from build123d import *

# Parameters (mm, degrees)
F0_R     = 2.50825
F1_DEPTH = 1.5875
F2_R     = 1.27


with BuildPart() as f1:
    # F0 (on Top) → F1 (new body)
    with BuildSketch(Plane.XY):
        with BuildLine():
            Line((2.667, 95.25), (0, 95.25))
            Line((0, 95.25), (-2.667, 95.25))
            ThreePointArc((-2.667, 95.25), (-3.5342102448, 94.8907897552), (-3.175, 95.758))
            Line((-3.175, 95.758), (-3.175, 114.3))
            Line((-3.175, 114.3), (-24.765, 114.3))
            Line((-24.765, 114.3), (-24.765, 0))
            Line((-24.765, 0), (-5.2613402643, -16.3655136908))
            ThreePointArc((-5.2613402643, -16.3655136908), (-3.9082748076, -16.5436481376), (-3.175, -15.3926372481))
            Line((-3.175, -15.3926372481), (-3.175, -0.508))
            ThreePointArc((-3.175, -0.508), (-3.5342102448, 0.3592102448), (-2.667, 0))
            Line((-2.667, 0), (0, 0))
            Line((0, 0), (2.667, 0))
            ThreePointArc((2.667, 0), (3.3487462328, 0.4773638514), (3.5641505771, -0.3265361057))
            ThreePointArc((3.5641505771, -0.3265361057), (3.389690077, -0.4604043558), (3.175, -0.508))
            Line((3.175, -0.508), (3.175, -15.3926372481))
            ThreePointArc((3.175, -15.3926372481), (3.9082748076, -16.5436481376), (5.2613402643, -16.3655136908))
            Line((5.2613402643, -16.3655136908), (24.765, 0))
            Line((24.765, 0), (24.765, 114.3))
            Line((24.765, 114.3), (3.175, 114.3))
            Line((3.175, 114.3), (3.175, 95.758))
            ThreePointArc((3.175, 95.758), (3.5342102448, 94.8907897552), (2.667, 95.25))
        make_face()
        with BuildLine():
            ThreePointArc((-3.683, 17.8998578738), (-3.175, 18.4078578738), (-2.667, 17.8998578738))
            Line((-2.667, 17.8998578738), (-2.667, 10.2798578738))
            ThreePointArc((-2.667, 10.2798578738), (-3.175, 9.7718578738), (-3.683, 10.2798578738))
            Line((-3.683, 10.2798578738), (-3.683, 17.8998578738))
        make_face(mode=Mode.SUBTRACT)
        with BuildLine():
            ThreePointArc((-3.683, 34.8687778738), (-3.175, 35.3767778738), (-2.667, 34.8687778738))
            Line((-2.667, 34.8687778738), (-2.667, 27.2487778738))
            ThreePointArc((-2.667, 27.2487778738), (-3.175, 26.7407778738), (-3.683, 27.2487778738))
            Line((-3.683, 27.2487778738), (-3.683, 34.8687778738))
        make_face(mode=Mode.SUBTRACT)
        with BuildLine():
            Line((-3.683, 44.2176978738), (-3.683, 51.8376978738))
            ThreePointArc((-3.683, 51.8376978738), (-3.175, 52.3456978738), (-2.667, 51.8376978738))
            Line((-2.667, 51.8376978738), (-2.667, 44.2176978738))
            ThreePointArc((-2.667, 44.2176978738), (-3.175, 43.7096978738), (-3.683, 44.2176978738))
        make_face(mode=Mode.SUBTRACT)
        with BuildLine():
            Line((3.683, 17.8998578738), (3.683, 10.2798578738))
            ThreePointArc((3.683, 10.2798578738), (3.175, 9.7718578738), (2.667, 10.2798578738))
            Line((2.667, 10.2798578738), (2.667, 17.8998578738))
            ThreePointArc((2.667, 17.8998578738), (3.175, 18.4078578738), (3.683, 17.8998578738))
        make_face(mode=Mode.SUBTRACT)
        with BuildLine():
            Line((3.683, 34.8687778738), (3.683, 27.2487778738))
            ThreePointArc((3.683, 27.2487778738), (3.175, 26.7407778738), (2.667, 27.2487778738))
            Line((2.667, 27.2487778738), (2.667, 34.8687778738))
            ThreePointArc((2.667, 34.8687778738), (3.175, 35.3767778738), (3.683, 34.8687778738))
        make_face(mode=Mode.SUBTRACT)
        with BuildLine():
            Line((3.683, 51.8376978738), (3.683, 44.2176978738))
            ThreePointArc((3.683, 44.2176978738), (3.175, 43.7096978738), (2.667, 44.2176978738))
            Line((2.667, 44.2176978738), (2.667, 51.8376978738))
            ThreePointArc((2.667, 51.8376978738), (3.175, 52.3456978738), (3.683, 51.8376978738))
        make_face(mode=Mode.SUBTRACT)
        with BuildLine():
            ThreePointArc((-3.683, 68.8048978738), (-3.175, 69.3128978738), (-2.667, 68.8048978738))
            Line((-2.667, 68.8048978738), (-2.667, 61.1848978738))
            ThreePointArc((-2.667, 61.1848978738), (-3.175, 60.6768978738), (-3.683, 61.1848978738))
            Line((-3.683, 61.1848978738), (-3.683, 68.8048978738))
        make_face(mode=Mode.SUBTRACT)
        with Locations((-12.7, 104.775)):
            Circle(F0_R, mode=Mode.SUBTRACT)
        with BuildLine():
            ThreePointArc((-3.683, 85.7720978738), (-3.175, 86.2800978738), (-2.667, 85.7720978738))
            Line((-2.667, 85.7720978738), (-2.667, 78.1520978738))
            ThreePointArc((-2.667, 78.1520978738), (-3.175, 77.6440978738), (-3.683, 78.1520978738))
            Line((-3.683, 78.1520978738), (-3.683, 85.7720978738))
        make_face(mode=Mode.SUBTRACT)
        with BuildLine():
            Line((3.683, 68.8048978738), (3.683, 61.1848978738))
            ThreePointArc((3.683, 61.1848978738), (3.175, 60.6768978738), (2.667, 61.1848978738))
            Line((2.667, 61.1848978738), (2.667, 68.8048978738))
            ThreePointArc((2.667, 68.8048978738), (3.175, 69.3128978738), (3.683, 68.8048978738))
        make_face(mode=Mode.SUBTRACT)
        with BuildLine():
            Line((3.683, 85.7720978738), (3.683, 78.1520978738))
            ThreePointArc((3.683, 78.1520978738), (3.175, 77.6440978738), (2.667, 78.1520978738))
            Line((2.667, 78.1520978738), (2.667, 85.7720978738))
            ThreePointArc((2.667, 85.7720978738), (3.175, 86.2800978738), (3.683, 85.7720978738))
        make_face(mode=Mode.SUBTRACT)
        with Locations((12.7, 104.775)):
            Circle(F0_R, mode=Mode.SUBTRACT)
    extrude(amount=F1_DEPTH)

    # F2
    f2_edges = [f1.edges().sort_by_distance(p)[0] for p in [
        (24.765, 0, 0.79375),
        (-24.765, 0, 0.79375),
        (-24.765, 114.3, 0.79375),
        (24.765, 114.3, 0.79375),
    ]]
    fillet(f2_edges, radius=F2_R)


solid = f1.part
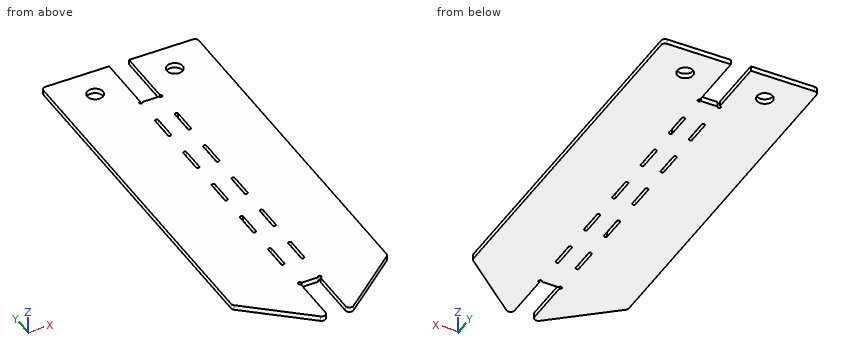
The listing builds one solid part. Answer for the finished solid, in the listing's coordinates (mm). Give positions to 0.01 mm unless a question says otherwise; leave off trailing zeros. Write each loop counter-clockwise with the first axis right and the second up, starting at its lowest first coordinate (ties: lowest second). Pieces come first, ordered by that corner, then holes.
1) Given P1, Ø6, axis at x = 12.7, y = 104.775, coming from the -Z side; P2, Ø0.9, axis at x = 3.175, y = 0, coming from the -Z side, each flat-ended and moving along its own axis, determine where each tip first touches the part or whether it passes through.
2) Section B-B (x = -12.7) is taken. Write down the section's boundary in (y, z), and give its area (3 significant figures).
3) Find the intervals of material crossed by L1, parallel to X at y = 85, z = 0.9 (3 decimals); L2, parallel to Y at x = -14, z = 0.9; L3, parallel to Y at x = 12, z = 0.55, in increasing order.
4) Section C-C (z = 0.85) is taken. Count the separate pieces of the cut face and the enclosed holes in it, and give its area (3 significant figures).
5) Section D-D (x = -21.5) is taken. Write down the section's boundary in (y, z).
6) Section A-A (y = 84) is taken. Write down the section's boundary in (x, z) (1 decimal), and give its area (3 significant figures).
Response:
1. P1: stops at z = 0
1. P2: passes through
2. outline: (-10.12, 0) - (102.27, 0) - (102.27, 1.59) - (-10.12, 1.59) - close; (107.28, 0) - (114.3, 0) - (114.3, 1.59) - (107.28, 1.59) - close
2. area: 190 mm2
3. L1: x = -24.765 to -3.683, -2.667 to 2.667, 3.683 to 24.765
3. L2: y = -9.03 to 102.63, 106.92 to 114.3
3. L3: y = -10.71 to 102.37, 107.18 to 114.3
4. separate pieces: 1
4. enclosed holes: 12
4. area: 5,800 mm2
5. outline: (-2.74, 0) - (114.3, 0) - (114.3, 1.59) - (-2.74, 1.59) - close
6. outline: (-24.8, 0) - (-3.7, 0) - (-3.7, 1.6) - (-24.8, 1.6) - close; (-2.7, 0) - (2.7, 0) - (2.7, 1.6) - (-2.7, 1.6) - close; (3.7, 0) - (24.8, 0) - (24.8, 1.6) - (3.7, 1.6) - close
6. area: 75.4 mm2
